Design review of the part built by this model. Coordinates are the model's own, in mm. Face numbers are marked on the shaded views. A direction names the side the tool comes from. Give positions to 0.01 mm unless a question says otherwise; leave off trailing zeros. Loops run counter-clockwise (first coordinate to the right, second up) from the corner with the lowest first, then second, coordinate; pieces in that order, holes last. Notation, with made-up numbers: M 41,-14.75 L 52,-14.75 A28 ccw 52,13.25 Z; hole C -38.5,-4.5 d9. An arc over 180 degrees is marked long. Answer as CSV lines item,"result".
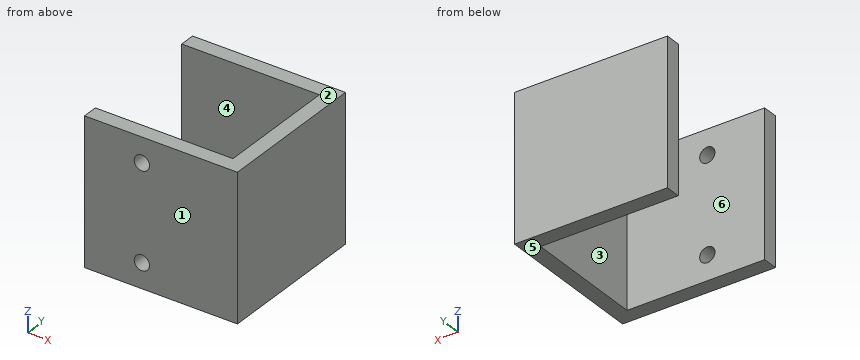
```python
from build123d import *

# Parameters (mm, degrees)
BOSS_EXTRU_1_DEPTH      = 38
ESQUISSE2_R             = 2
ENL_V_MAT_EXTRU_1_DEPTH = 10


with BuildPart() as part:
    # Esquisse1 → Boss.-Extru.1 (new body)
    with BuildSketch(Plane.XY):
        Polygon((16, 34), (16, 18), (20, 18), (20, 38), (-20, 38), (-20, 34), align=None)
        Polygon((-20, 2), (-20, -2), (13.980877288, -2), (20, -2), (20, 2), (20, 18), (16, 18), (16, 2), align=None)
    extrude(amount=BOSS_EXTRU_1_DEPTH)

    # Esquisse2 → Enlèv. mat.-Extru.1 (cut)
    with BuildSketch(Plane.XZ.offset(2)):
        with Locations((-5, 31.5)):
            Circle(ESQUISSE2_R)
        with Locations((-5, 6.5)):
            Circle(ESQUISSE2_R)
    extrude(amount=-ENL_V_MAT_EXTRU_1_DEPTH, mode=Mode.SUBTRACT)


solid = part.part
```
1. We need section C-C, the plane x = -17. Write out the cut boundary in (y, z), plus the area to 3 significant figures.
Answer block:
outline,"M -2,0 L 2,0 L 2,38 L -2,38 Z; M 34,0 L 38,0 L 38,38 L 34,38 Z"
area,"304 mm²"
2. For P1, Ø6, axis at y = 15.5, z = 18.5, coming from the -X side, flat-tipped, find the tip position at first contact; note if it passes through.
Answer block:
P1,"x = 16"
3. The part is to be moulded in two halves that separate along Y. For the marked faces 1, 2, 3 and 4, say which applies: pulls with the +Y half, pulls with the -Y half, needs draft (parallel to the pull), parting line crosses it, or undercut.
Answer block:
face 1,"pulls with the -Y half"
face 2,"needs draft"
face 3,"undercut"
face 4,"undercut"
4. We need section A-A, the plane x = -5. Write out the cut boundary in (y, z).
Answer block:
outline,"M -2,0 L 2,0 L 2,4.5 L -2,4.5 Z; M -2,8.5 L 2,8.5 L 2,29.5 L -2,29.5 Z; M -2,33.5 L 2,33.5 L 2,38 L -2,38 Z; M 34,0 L 38,0 L 38,38 L 34,38 Z"
5. For the marked faces 5 and 6, list the 3-axis set-ups (+Z, -Z, +X, -X, +Y, -Y) from which the entire face can be reached by the end or side of a thin tool; tool diameter is ignored.
Answer block:
face 5,"-Z, +X, -X, +Y, -Y"
face 6,"+Z, -Z, -X"
6. We need section B-B, the plane z = 31.5. Write out the cut boundary in (x, y), plus the area to 3 significant figures.
Answer block:
outline,"M -20,-2 L -7,-2 L -7,2 L -20,2 Z; M -20,34 L 16,34 L 16,2 L -3,2 L -3,-2 L 20,-2 L 20,38 L -20,38 Z"
area,"432 mm²"
7. We need section D-D, the plane z = 22. Write out the cut boundary in (x, y).
Answer block:
outline,"M -20,-2 L 20,-2 L 20,38 L -20,38 L -20,34 L 16,34 L 16,2 L -20,2 Z"
8. To check wall thickness, follow L1, parallel to Z at x = -5, y = 0.8; L2, parallel to Y at x = 5, z = 21; L3, parallel to X at y = 7.5, z = 18. State the ranges of each line that lie inside material, in increasing order. Write a range as [from, to].
Answer block:
L1,"[0, 4.5], [8.5, 29.5], [33.5, 38]"
L2,"[-2, 2], [34, 38]"
L3,"[16, 20]"
